from build123d import *

# Parameters (mm, degrees)
CENTER_MC_BODY_DEPTH           = 9.525
SKETCH2_R                      = 3.9624
CENTER_MC_HOLE_DEPTH           = 9.525
SKETCH3_W                      = 19.05
SKETCH3_H                      = 6.35
SKETCH3_W_2                    = 25.4
CUT_SLOT_DEPTH                 = 9.525
FILLET1_R                      = 12.7
FILLET2_R                      = 12.7
SKETCH12_W                     = 99.695
SKETCH12_H                     = 25.4
CUT_EXTRUDE2_DEPTH             = 10.5250001
BOSS_EXTRUDE1_DEPTH            = 9.525
FILLET3_R                      = 3.175
SKETCH14_W                     = 22.86
SKETCH14_H                     = 27.94
SKETCH14_R                     = 4.7117
BOSS_EXTRUDE2_DEPTH            = 9.525
SKETCH16_W                     = 53.975
SKETCH16_H                     = 15.24
CUT_FOR_THROTTLE_N_BRAKE_DEPTH = 9.525
SKETCH17_W                     = 58.42
SKETCH17_H                     = 48.26
SKETCH17_R                     = 4.7117
BOSS_EXTRUDE3_DEPTH            = 9.525
SKETCH44_W                     = 58.42
SKETCH44_H                     = 48.26
SKETCH44_R                     = 4.7117
BOSS_EXTRUDE4_DEPTH            = 25.4
SKETCH20_R                     = 2.413
CUT_EXTRUDE6_DEPTH             = 35.925
SKETCH21_R                     = 2.413
CUT_EXTRUDE7_DEPTH             = 35.925
CIRPATTERN2_COUNT              = 5
CIRPATTERN2_ANGLE              = 120
SKETCH22_R                     = 2.413
CUT_EXTRUDE10_DEPTH            = 35.925
CIRPATTERN3_COUNT              = 5
CIRPATTERN3_ANGLE              = 120
SKETCH24_R                     = 2.413
CUT_EXTRUDE11_DEPTH            = 35.925
CIRPATTERN4_COUNT              = 4
CIRPATTERN4_ANGLE              = 90
SKETCH48_W                     = 22.225
SKETCH48_H                     = 107.218507126
CUT_EXTRUDE24_DEPTH            = 38.1
SKETCH49_W                     = 22.225
SKETCH49_H                     = 35.56
CUT_EXTRUDE25_DEPTH            = 21.32
FILLET4_R                      = 12.7
FILLET5_R                      = 33.02
FILLET6_R                      = 13.97
SKETCH53_R                     = 2.413
CUT_EXTRUDE29_DEPTH            = 35.925
FILLET7_R                      = 2.54


with BuildPart() as part:
    # Sketch1 → Center MC Body (new body)
    with BuildSketch(Plane(origin=(0, 0, 0), x_dir=(0, 0, -1), z_dir=(1, 0, 0))):
        with BuildLine():
            Line((-12.7, 0), (-12.7, 15.24))
            Line((-12.7, 15.24), (138.43, 15.24))
            Line((138.43, 15.24), (138.43, 16.51))
            ThreePointArc((138.43, 16.51), (147.32, 25.4), (156.21, 16.51))
            Line((156.21, 16.51), (156.21, 0))
            Line((156.21, 0), (-12.7, 0))
        make_face()
    extrude(amount=CENTER_MC_BODY_DEPTH)

    # Sketch2 → Center MC Hole (cut)
    with BuildSketch(Plane(origin=(0, 0, 0), x_dir=(0, 0, -1), z_dir=(1, 0, 0))):
        with Locations((147.32, 16.51)):
            Circle(SKETCH2_R)
    extrude(amount=CENTER_MC_HOLE_DEPTH, mode=Mode.SUBTRACT)

    # Sketch3 → Cut Slot (cut)
    with BuildSketch(Plane(origin=(0, 0, 0), x_dir=(0, 0, -1), z_dir=(1, 0, 0))):
        with Locations((3.175, 12.065)):
            Rectangle(SKETCH3_W, SKETCH3_H)
        with Locations((56.515, 12.065)):
            Rectangle(SKETCH3_W_2, SKETCH3_H)
    extrude(amount=CUT_SLOT_DEPTH, mode=Mode.SUBTRACT)

    # Fillet1
    fillet1_edges = [part.edges().sort_by_distance(p)[0] for p in [
        (4.7625, 0, -156.21),
    ]]
    fillet(fillet1_edges, radius=FILLET1_R)

    # Fillet2
    fillet2_edges = [part.edges().sort_by_distance(p)[0] for p in [
        (4.7625, 15.24, -138.43),
    ]]
    fillet(fillet2_edges, radius=FILLET2_R)

    # Sketch12 → Cut-Extrude2 (cut, through all)
    with BuildSketch(Plane(origin=(0, 0, 0), x_dir=(0, 0, -1), z_dir=(1, 0, 0))):
        with Locations((106.3625, 12.7)):
            Rectangle(SKETCH12_W, SKETCH12_H)
    extrude(amount=CUT_EXTRUDE2_DEPTH, mode=Mode.SUBTRACT)

    # Sketch13 → Boss-Extrude1 (add)
    with BuildSketch(Plane(origin=(0, 0, 0), x_dir=(0, 0, -1), z_dir=(1, 0, 0))):
        Polygon((43.815, 15.24), (50.165, 15.24), (50.165, 8.89), (62.865, 8.89), (62.865, 15.24), (66.675, 15.24), (66.675, 0), (43.815, 0), align=None)
    extrude(amount=BOSS_EXTRUDE1_DEPTH)

    # Fillet3
    fillet3_edges = [part.edges().sort_by_distance(p)[0] for p in [
        (4.7625, 15.24, -66.675),
        (4.7625, 0, -66.675),
    ]]
    fillet(fillet3_edges, radius=FILLET3_R)

    # Sketch14 → Boss-Extrude2 (add)
    with BuildSketch(Plane(origin=(0, 0, 0), x_dir=(0, 0, -1), z_dir=(1, 0, 0))):
        with Locations((-24.13, 13.97)):
            Rectangle(SKETCH14_W, SKETCH14_H)
        with Locations((-22.86, 16.51)):
            Circle(SKETCH14_R, mode=Mode.SUBTRACT)
    extrude(amount=BOSS_EXTRUDE2_DEPTH)

    # Sketch16 → Cut for Throttle n Brake (cut)
    with BuildSketch(Plane(origin=(0, 0, 0), x_dir=(0, 0, -1), z_dir=(1, 0, 0))):
        with Locations((39.6875, 7.62)):
            Rectangle(SKETCH16_W, SKETCH16_H)
    extrude(amount=CUT_FOR_THROTTLE_N_BRAKE_DEPTH, mode=Mode.SUBTRACT)

    # Sketch17 → Boss-Extrude3 (add)
    with BuildSketch(Plane(origin=(0, 0, 0), x_dir=(0, 0, -1), z_dir=(1, 0, 0))):
        with Locations((-16.51, 24.13)):
            Rectangle(SKETCH17_W, SKETCH17_H)
        with Locations((-22.86, 16.51)):
            Circle(SKETCH17_R, mode=Mode.SUBTRACT)
    extrude(amount=BOSS_EXTRUDE3_DEPTH)

    # Sketch44 → Boss-Extrude4 (add)
    with BuildSketch(Plane(origin=(9.525, 0, 0), x_dir=(0, 0, -1), z_dir=(1, 0, 0))):
        with Locations((-16.51, 24.13)):
            Rectangle(SKETCH44_W, SKETCH44_H)
        with Locations((-22.86, 16.51)):
            Circle(SKETCH44_R, mode=Mode.SUBTRACT)
    extrude(amount=BOSS_EXTRUDE4_DEPTH)

    # Sketch20 → Cut-Extrude6 (cut, through all)
    with BuildSketch(Plane(origin=(0, 0, 0), x_dir=(0, 0, -1), z_dir=(1, 0, 0))):
        with Locations((-40.64, 16.51)):
            Circle(SKETCH20_R)
    extrude(amount=CUT_EXTRUDE6_DEPTH, mode=Mode.SUBTRACT)

    # Sketch21 → Cut-Extrude7 (cut, through all)
    with BuildSketch(Plane(origin=(0, 0, 0), x_dir=(0, 0, -1), z_dir=(1, 0, 0))):
        with Locations((-40.457636205, 26.67)):
            Circle(SKETCH21_R)
    cut_extrude7 = extrude(amount=CUT_EXTRUDE7_DEPTH, mode=Mode.SUBTRACT)

    # CirPattern2: Cut-Extrude7 ×5 about axis
    cirpattern2_axis = Axis((0, 16.51, 22.86), (-1, 0, 0))
    for i in range(1, CIRPATTERN2_COUNT):
        add(cut_extrude7.rotate(cirpattern2_axis, i * CIRPATTERN2_ANGLE / (CIRPATTERN2_COUNT - 1)), mode=Mode.SUBTRACT)

    # Sketch22 → Cut-Extrude10 (cut, through all)
    with BuildSketch(Plane(origin=(0, 0, 0), x_dir=(0, 0, -1), z_dir=(1, 0, 0))):
        with Locations((-40.371499436, 34.021499436)):
            Circle(SKETCH22_R)
    cut_extrude10 = extrude(amount=CUT_EXTRUDE10_DEPTH, mode=Mode.SUBTRACT)

    # CirPattern3: Cut-Extrude10 ×5 about axis
    cirpattern3_axis = Axis((0, 16.51, 22.86), (-1, 0, 0))
    for i in range(1, CIRPATTERN3_COUNT):
        add(cut_extrude10.rotate(cirpattern3_axis, i * CIRPATTERN3_ANGLE / (CIRPATTERN3_COUNT - 1)), mode=Mode.SUBTRACT)

    # Sketch24 → Cut-Extrude11 (cut, through all)
    with BuildSketch(Plane(origin=(0, 0, 0), x_dir=(0, 0, -1), z_dir=(1, 0, 0))):
        with Locations((-36.83, 40.706749782)):
            Circle(SKETCH24_R)
    cut_extrude11 = extrude(amount=CUT_EXTRUDE11_DEPTH, mode=Mode.SUBTRACT)

    # CirPattern4: Cut-Extrude11 ×4 about axis
    cirpattern4_axis = Axis((0, 16.51, 22.86), (-1, 0, 0))
    for i in range(1, CIRPATTERN4_COUNT):
        add(cut_extrude11.rotate(cirpattern4_axis, i * CIRPATTERN4_ANGLE / (CIRPATTERN4_COUNT - 1)), mode=Mode.SUBTRACT)

    # Sketch48 → Cut-Extrude24 (cut)
    with BuildSketch(Plane.XY.offset(45.72)):
        with Locations((17.4625, 53.609253563)):
            Rectangle(SKETCH48_W, SKETCH48_H)
    extrude(amount=-CUT_EXTRUDE24_DEPTH, mode=Mode.SUBTRACT)

    # Sketch49 → Cut-Extrude25 (cut, through all)
    with BuildSketch(Plane.XY.offset(7.62)):
        with Locations((17.4625, 30.48)):
            Rectangle(SKETCH49_W, SKETCH49_H)
    extrude(amount=-CUT_EXTRUDE25_DEPTH, mode=Mode.SUBTRACT)

    # Fillet4
    fillet4_edges = [part.edges().sort_by_distance(p)[0] for p in [
        (31.75, 0, 45.72),
        (3.175, 0, 45.72),
    ]]
    fillet(fillet4_edges, radius=FILLET4_R)

    # Fillet5
    fillet5_edges = [part.edges().sort_by_distance(p)[0] for p in [
        (31.75, 48.26, -12.7),
        (3.175, 48.26, -12.7),
    ]]
    fillet(fillet5_edges, radius=FILLET5_R)

    # Fillet6
    fillet6_edges = [part.edges().sort_by_distance(p)[0] for p in [
        (31.75, 48.26, 45.72),
        (3.175, 48.26, 45.72),
    ]]
    fillet(fillet6_edges, radius=FILLET6_R)

    # Sketch53 → Cut-Extrude29 (cut, through all)
    with BuildSketch(Plane(origin=(34.925, 0, 0), x_dir=(0, 0, -1), z_dir=(1, 0, 0))):
        with Locations((2.54, 6.35)):
            Circle(SKETCH53_R)
    extrude(amount=-CUT_EXTRUDE29_DEPTH, mode=Mode.SUBTRACT)

    # Fillet7
    fillet7_edges = [part.edges().sort_by_distance(p)[0] for p in [
        (17.4625, 0, -12.7),
    ]]
    fillet(fillet7_edges, radius=FILLET7_R)


solid = part.part
Input: part model. Units: mm. Frame: model coordinates. Give positions to 0.01 mm unless a question says otherwise; leave off trailing zeros. Order: outer loops, then holes, each group sorted by start corner. A loop starts at its lowest first (then second) coordinate and runs counter-clockwise, first axis right, second up.
Q1. Section C-C on z = 8.89. Output: boundary loops of the cut face in (x, y) (3 decimals).
Checked values:
outline: (0, 0) - (6.35, 0) - (6.35, 38.294) - (0, 38.294) - close; (0, 43.12) - (6.35, 43.12) - (6.35, 46.219) - (0, 46.219) - close; (28.575, 0) - (34.925, 0) - (34.925, 38.294) - (28.575, 38.294) - close; (28.575, 43.12) - (34.925, 43.12) - (34.925, 46.219) - (28.575, 46.219) - close
Q2. Contact query for flat-ended pins moving along their axis: pin 1 Ø8 at (x, y) = (4, 31) entering from -Z; pin 2 Ø14 at (x, y) = (16, 8) entering from +Z. Output: stop coordinate, or through.
Checked values:
pin 1: stops at z = -10.53
pin 2: stops at z = 7.62
Q3. Section B-B on y = 16.51. Output: boundary loops of the cut face in (x, z) (3 decimals), and give its area (3 significant figures).
Checked values:
outline: (0, -12.676) - (6.35, -12.676) - (6.35, 18.148) - (0, 18.148) - close; (0, 27.572) - (6.35, 27.572) - (6.35, 38.227) - (0, 38.227) - close; (0, 43.053) - (6.35, 43.053) - (6.35, 45.72) - (0, 45.72) - close; (28.575, -12.676) - (34.925, -12.676) - (34.925, 18.148) - (28.575, 18.148) - close; (28.575, 27.572) - (34.925, 27.572) - (34.925, 38.227) - (28.575, 38.227) - close; (28.575, 43.053) - (34.925, 43.053) - (34.925, 45.72) - (28.575, 45.72) - close
area: 561 mm2
Q4. Section A-A on x = 14.5. Output: boundary loops of the cut face in (y, z).
Checked values:
outline: (0, -10.16) arc R2.54 ccw to (2.54, -12.7) - (12.7, -12.7) - (12.7, 7.62) - (0, 7.62) - close; hole circle Ø4.83 at (6.35, -2.54)
Q5. Draft query along Z for faces 1 (the cylindrical face through (3.22, 3.82, 42.1)), 2 (the flat face through (17, 9, -12.7)), 3 (the cylindrical face through (31.706, 38.971, 23.973)). Return one class per face: +Z half, -Z half, draft (parallel to the pull), parting line (faces both ways), or undercut.
Checked values:
face 1: +Z half
face 2: -Z half
face 3: undercut
Q6. Section D-D on y = 45.5. Output: boundary loops of the cut face in (x, z) (3 decimals).
Checked values:
outline: (0, 7.104) - (6.35, 7.104) - (6.35, 20.687) - (0, 20.687) - close; (0, 25.033) - (6.35, 25.033) - (6.35, 40.086) - (0, 40.086) - close; (28.575, 7.104) - (34.925, 7.104) - (34.925, 20.687) - (28.575, 20.687) - close; (28.575, 25.033) - (34.925, 25.033) - (34.925, 40.086) - (28.575, 40.086) - close
Q7. Ray query, probe 1 along Y at (x, z) = (5.25, 22.86); probe 2 along X at (y, z) = (5, 29) (3 decimals); probe 3 along Y at (x, z) = (4.5, 0.5). Return the intervals inside material, ascending.
Checked values:
probe 1: y = 0 to 11.8, 21.22 to 34.42, 39.24 to 42.04, 46.86 to 48.26
probe 2: x = 0 to 6.35, 28.575 to 34.925
probe 3: y = 0 to 21.08, 24.76 to 28.92, 32.04 to 41.65
